Check sheet for the modelled part. Datum: model origin and axes. Units: mm. Give positions to 0.01 mm unless a question says otherwise; leave off trailing zeros. Write each loop counter-clockwise with the first axis right and the second up, starting at its lowest first coordinate (ties: lowest second). Pieces come first, ordered by that corner, then holes. Notation, with made-up numbers: (49.25, 10.5) -> (86.25, 10.5) arc R26 cw to (86.25, 36.5) -> close; hole circle Ø3 at (-34.75, -20.5). An arc over 180 degrees is marked (long way). Use a Markdown table: item, result. Add a question column.
1. Cross-section at B-B (y = -83). Enter the section's corners in (x, z), then the cut area to 3 significant figures.
2. Cross-section at A-A (z = 2.3). Count the separate pieces of the cut face and the enclosed holes in it, then the cut area to 3 significant figures.
3. Scan lines: probe 1 along X at (y, z) = (-55, 4.7); probe 2 along Y at (x, z) = (-8, 3); probe 3 along Y at (x, z) = (9.75, 3.4). Record each from-to range of solid material in increasing order. Write a range as [from, to].
4. Gauge pin test, flat ends, axial feed: P1, Ø1.5, axis at y = -10, z = 1, coming from the +X side; P2, Ø1.5, axis at x = -3.5, z = 2, coming from the -Y side. Record the tip position at first contact, or that the pin passes through.
Autodesk Inventor part; units mm, degrees
ref_plane "YZ Plane" through (0, 0, 0) normal (1, 0, 0) x (0, 1, 0)
ref_plane "XZ Plane" through (0, 0, 0) normal (0, 1, 0) x (-1, 0, 0)
ref_plane "XY Plane" through (0, 0, 0) normal (0, 0, 1) x (1, 0, 0)
sketch "Esquisse4" plane through (0, 0, 0) normal (0, 0, 1) x (1, 0, 0)
  line L0 (0, 0) -> (9, 0)
  line L1 (9, 0) -> (9, -7.36)
  line L2 (9, -7.36) -> (13, -7.36)
  line L3 (13, -7.36) -> (13, -122.36)
  line L4 (13, -122.36) -> (-4, -122.36)
  line L5 (-4, -122.36) -> (-4, -7.36)
  line L6 (-4, -7.36) -> (0, -7.36)
  line L7 (0, -7.36) -> (0, 0)
  arc A0 (-4, -122.36) -> (13, -122.36) centre (4.5, -120.3919) ccw
  line L8 (-9.0237, 0) -> (15.6194, 0)
  line L9 (15.6194, 0) -> (15.6194, 7.3414)
  line L10 (15.6194, 7.3414) -> (-9.0237, 7.3414)
  line L11 (-9.0237, 7.3414) -> (-9.0237, 0)
  dimension "d8" = 4
  dimension "d9" = 4
  dimension "d10" = 9
  dimension "d11" = 115
  dimension "d12" = 24.6431
extrude "Extrusion1" add sketch "Esquisse4" along normal blind 5
fillet "Congé1" radius 2 2 edges at (13, -7.36, 2.5) (-4, -7.36, 2.5)
hole "Perçage1" at (4.6143, -119.075, 0) direction (0, 0, 1) diameter 0.5 end through all
pattern_linear "Réseau rectangulaire1" count 10 spacing 10 along (0, 1, 0) of "Perçage1"
sketch "Esquisse5" plane through (0, 0, 0) normal (0, 0, -1) x (-1, 0, 0)
  point P0 (0, 0)
properties part number "bracelet" material "Caoutchouc"
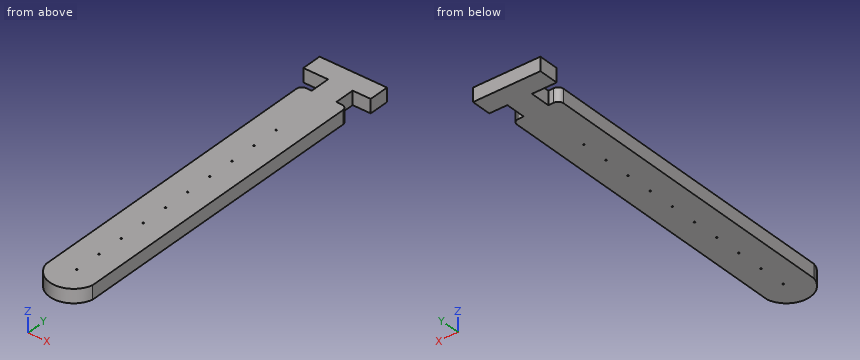
Worked answers:
| question | item | result |
|---|---|---|
| 1 | outline | (-4, 0) -> (13, 0) -> (13, 5) -> (-4, 5) -> close |
| 1 | area | 85.0 mm² |
| 2 | separate pieces | 1 |
| 2 | enclosed holes | 10 |
| 2 | area | 2,280 mm² |
| 3 | probe 1 | x = [-4, 13] |
| 3 | probe 2 | y = [0, 7.34] |
| 3 | probe 3 | y = [-127.36, -7.36], [0, 7.34] |
| 4 | P1 | stops at x = 13 |
| 4 | P2 | stops at y = -125.25 |
